Check sheet for the modelled part. Datum: model origin and axes. Units: mm. A direction names the side the tool comes from. Coordinates: 2 decimals unless noted, no trailing zeros. Write each loop counter-clockwise with the first axis right and the second up, starting at its lowest first coordinate (ties: lowest second). Pieces come first, ordered by that corner, then holes. Notation, with made-up numbers: M 59.5,11 L 102.5,11 A33 ccw 102.5,41 Z; hole C 29.25,-20 d10. An arc over 180 degrees is marked long. Answer as CSV lines item,"result". Start each with the question number.
1) Section check D-D (y = 71). Record the cut outline in (x, z), and give its area (3 significant figures).
2) Go/stop test with flat-tipped pins: pin 1 Ø14.5 at (x, y) = (-1.5, 18.5) entering from +Z; pin 2 Ø2.5 at (x, z) = (0, 13.5) entering from +Y; pin 3 Ø2.5 at (x, z) = (0, -14) entering from +Y. Record where each tip stops, or that it passes through.
3) Access from +Z, -Z, +X, -X, +Y, -Y to the whole of each face (thin tool, end or side, straight path). Record for faces 5 (the flat face through (0, 22, 20.5)), 6 (the flat face through (0, 0, 0)), 7 (the flat face through (18.179, 21.797, 18.113)), 8 (the flat face through (-19, 44, 0)).
4) Draft check along X on faces 1 (the flat face through (0, 22, -20.5)), 2 (the flat face through (0, 58, -14)), 3 (the flat face through (-21, 40, 0)), 4 (the flat face through (0, 58, 14)). Enter one of: +X half, -X half, draft (parallel to the pull), parting line (faces both ways), or undercut.
5) Material ranges on L1, parallel to Z at x = 1, y = 28; L2, parallel to Y at x = 10, z = 12.5; L3, parallel to X at y = 62, z = 14, recorded low to high. Write a range as [from, to].
6) Section check A-A (y = 24). Record the cut outline in (x, z).
from build123d import *

# Parameters (mm, degrees)
SKETCH1_W           = 42
SKETCH1_H           = 42
BOSS_EXTRUDE1_DEPTH = 44
SKETCH2_R           = 18
BOSS_EXTRUDE2_DEPTH = 24
SKETCH3_R           = 4
BOSS_EXTRUDE3_DEPTH = 18
CHAMFER1_SIZE       = 5
SKETCH4_R           = 1.5
CUT_EXTRUDE1_DEPTH  = 10
CIRPATTERN1_COUNT   = 4
CHAMFER2_SIZE       = 1
CUT_EXTRUDE2_START  = -7.5
CUT_EXTRUDE2_DEPTH  = 29
CHAMFER4_SIZE       = 0.5


with BuildPart() as part:
    # Sketch1 → Boss-Extrude1 (new body)
    with BuildSketch(Plane(origin=(0, 0, 0), x_dir=(1, 0, 0), z_dir=(0, 1, 0))):
        Rectangle(SKETCH1_W, SKETCH1_H)
    extrude(amount=BOSS_EXTRUDE1_DEPTH)

    # Sketch2 → Boss-Extrude2 (add)
    with BuildSketch(Plane(origin=(0, 44, 0), x_dir=(1, 0, 0), z_dir=(0, 1, 0))):
        with Locations(Location((0, 0, 0), (0, 0, 270))):
            Circle(SKETCH2_R)
    extrude(amount=BOSS_EXTRUDE2_DEPTH)

    # Sketch3 → Boss-Extrude3 (add)
    with BuildSketch(Plane(origin=(0, 68, 0), x_dir=(1, 0, 0), z_dir=(0, 1, 0))):
        with Locations(Location((0, 0, 0), (0, 0, 270))):
            Circle(SKETCH3_R)
    extrude(amount=BOSS_EXTRUDE3_DEPTH)

    # Chamfer1
    chamfer1_edges = [part.edges().sort_by_distance(p)[0] for p in [
        (21, 22, 21),
        (-21, 22, 21),
        (-21, 22, -21),
        (21, 22, -21),
    ]]
    chamfer(chamfer1_edges, length=CHAMFER1_SIZE)

    # Sketch4 → Cut-Extrude1 (cut)
    with BuildSketch(Plane(origin=(0, 68, 0), x_dir=(1, 0, 0), z_dir=(0, 1, 0))):
        with Locations(Location((0, 14, 0), (0, 0, 270))):
            Circle(SKETCH4_R)
    cut_extrude1 = extrude(amount=-CUT_EXTRUDE1_DEPTH, mode=Mode.SUBTRACT)

    # CirPattern1: Cut-Extrude1 ×4 about axis
    cirpattern1_axis = Axis((0, 0, 0), (0, 1, 0))
    for i in range(1, CIRPATTERN1_COUNT):
        add(cut_extrude1.rotate(cirpattern1_axis, i * 360 / CIRPATTERN1_COUNT), mode=Mode.SUBTRACT)

    # Chamfer2
    chamfer2_edges = [part.edges().sort_by_distance(p)[0] for p in [
        (0, 68, -18),
    ]]
    chamfer(chamfer2_edges, length=CHAMFER2_SIZE)

    # Sketch5 → Cut-Extrude2 (cut)
    with BuildSketch(Plane.XZ.offset(CUT_EXTRUDE2_START)):
        Polygon((-21, 16), (-21, -16), (-16, -21), (16, -21), (21, -16), (21, 16), (16, 21), (-16, 21), align=None)
        Polygon((-20.5, 15.792893219), (-20.5, -15.792893219), (-15.792893219, -20.5), (15.792893219, -20.5), (20.5, -15.792893219), (20.5, 15.792893219), (15.792893219, 20.5), (-15.792893219, 20.5), align=None, mode=Mode.SUBTRACT)
    extrude(amount=-CUT_EXTRUDE2_DEPTH, mode=Mode.SUBTRACT)

    # Chamfer4
    chamfer4_edges = [part.edges().sort_by_distance(p)[0] for p in [
        (-21, 0, 0),
        (-21, 44, 0),
        (21, 0, 0),
        (0, 0, 21),
        (0, 0, -21),
        (-18.5, 0, 18.5),
        (18.5, 0, 18.5),
        (18.5, 0, -18.5),
        (-18.5, 0, -18.5),
        (0, 44, -21),
        (21, 44, 0),
        (0, 44, 21),
        (-18.5, 44, 18.5),
        (18.5, 44, 18.5),
        (18.5, 44, -18.5),
        (-18.5, 44, -18.5),
    ]]
    chamfer(chamfer4_edges, length=CHAMFER4_SIZE)


solid = part.part
Results found:
1,outline,"C 0,0 d8"
1,area,"50.3 mm2"
2,pin 1,"stops at z = 20.5"
2,pin 2,"stops at y = 68"
2,pin 3,"stops at y = 58"
3,face 5,"+Z, +X, -X"
3,face 6,"+Z, -Z, +X, -X, -Y"
3,face 7,"+Z, +X"
3,face 8,"+Y"
4,face 1,"draft"
4,face 2,"undercut"
4,face 3,"-X half"
4,face 4,"undercut"
5,L1,"z = [-20.5, 20.5]"
5,L2,"y = [0, 68]"
5,L3,"x = [-11.31, -1.5], [1.5, 11.31]"
6,outline,"M -20.5,-15.79 L -15.79,-20.5 L 15.79,-20.5 L 20.5,-15.79 L 20.5,15.79 L 15.79,20.5 L -15.79,20.5 L -20.5,15.79 Z"
